Check sheet for the modelled part. Datum: model origin and axes. Units: mm. Give positions to 0.01 mm unless a question says otherwise; leave off trailing zeros. Loops run counter-clockwise (first coordinate to the right, second up) from the corner with the lowest first, then second, coordinate; pieces in that order, holes last. Notation, with made-up numbers: M 20,13.5 L 72,13.5 A10 cw 72,30.5 Z; hole C 35.25,7 d7. An arc over 180 degrees is marked long. Use one line per item in the form item = value.
from build123d import *

# Parameters (mm, degrees)
F0_W           = 152.4
F0_H           = 76.2
F1_DEPTH       = 3.175
F3_D           = 3.175
F3_CSINK_D     = 6.35
F3_CSINK_ANGLE = 82


# Not quite as in the source:
# - a feature names something its author has since deleted; it is built from what else it names


with BuildPart() as f1:
    # F0 (on Top) → F1 (new body)
    with BuildSketch(Plane.XY):
        with Locations((76.2, 38.1)):
            Rectangle(F0_W, F0_H)
    extrude(amount=F1_DEPTH)

    # F3 (through all)
    with Locations(Plane(origin=(0, 0, 0), x_dir=(1, 0, 0), z_dir=(0, 0, -1))):
        with Locations((3.81, -3.81), (3.81, -36.83), (3.81, -72.39), (148.59, -72.39), (148.59, -39.37), (148.59, -457.2), (76.2, -3.81), (76.2, -72.39), (148.9000022411, -3.81)):
            CounterSinkHole(F3_D / 2, F3_CSINK_D / 2, counter_sink_angle=F3_CSINK_ANGLE)


solid = f1.part
1) Release check for a two-part mould opening along Y. For faces 1 (the face through (0, 38, 2)), 2 (the face through (75, 0, 2)), 3 (the face through (4.98, 35.757, 2.51)), 4 (the face through (147.386, 3.333, 2.51)) record: pulls with the +Y half, pulls with the -Y half, needs draft (parallel to the pull), parting line crosses it, or undercut.
Evaluation:
face_1 = needs draft
face_2 = pulls with the -Y half
face_3 = undercut
face_4 = undercut
2) Depth check by flat-ended pin: pin 1 Ø3.5 at (x, y) = (3.81, 3.81) entering from -Z. Enter the tip coordinate at first touch or a pass-through.
Evaluation:
pin_1 = 1.64
3) Scan lines: line 1 (Y direction, x = 3.81, z = 2.25); line 2 (X direction, y = 72.39, z = 2.3); line 3 (Y direction, x = 76.2, z = 2.65). Record each from-to range of solid material in increasing order.
Evaluation:
line_1 = 0 to 2.22, 5.4 to 35.24, 38.42 to 70.8, 73.98 to 76.2
line_2 = 0 to 2.22, 5.4 to 74.61, 77.79 to 147, 150.18 to 152.4
line_3 = 0 to 2.22, 5.4 to 70.8, 73.98 to 76.2
4) Section check B-B (y = 3.81). State how many separate pieces and enclosed holes the cut face has, then the cut area to 3 significant figures.
Evaluation:
separate_pieces = 4
enclosed_holes = 0
area = 445 mm^2
5) Section check A-A (x = 3.81). Record the cut outline in (y, z) (1 decimal), then the cut area to 3 significant figures.
Evaluation:
outline = M 0,0 L 0.6,0 L 2.2,1.8 L 2.2,3.2 L 0,3.2 Z; M 5.4,1.8 L 7,0 L 33.7,0 L 35.2,1.8 L 35.2,3.2 L 5.4,3.2 Z; M 38.4,1.8 L 40,0 L 69.2,0 L 70.8,1.8 L 70.8,3.2 L 38.4,3.2 Z; M 74,1.8 L 75.6,0 L 76.2,0 L 76.2,3.2 L 74,3.2 Z
area = 203 mm^2
